from build123d import *

# Parameters (mm, degrees)
SKETCH_1_W           = 40
SKETCH_1_H           = 40
EXTRUDE_1_DEPTH      = 8
SKETCH_2_W           = 8
SKETCH_2_H           = 40
CUT_EXTRUDE_1_DEPTH  = 3.5
SKETCH_3_R           = 1.15
CUT_EXTRUDE_2_DEPTH  = 58.131427428
SKETCH_4_R           = 2
CUT_EXTRUDE_3_DEPTH  = 2.4
SKETCH_5_W           = 14.5
SKETCH_5_H           = 16
CUT_EXTRUDE_4_DEPTH  = 4
FILLET_2_R           = 0.5
SKETCH_6_W           = 1.5
SKETCH_6_H           = 1.5
CUT_EXTRUDE_5_DEPTH  = 4
SKETCH_7_R           = 1
CUT_EXTRUDE_6_DEPTH  = 4
FILLET_3_R           = 0.75
FILLET_4_R           = 0.75
CUT_EXTRUDE_7_DEPTH  = 4
SKETCH_10_R          = 3.6
CUT_EXTRUDE_9_DEPTH  = 4.5
SKETCH_11_R          = 2.1
CUT_EXTRUDE_10_DEPTH = 57.747246629


with BuildPart() as part:
    # 草图1 → 凸台-拉伸1 (new body)
    with BuildSketch(Plane(origin=(0, 0, 0), x_dir=(1, 0, 0), z_dir=(0, 1, 0))):
        with Locations((20, -20)):
            Rectangle(SKETCH_1_W, SKETCH_1_H)
    extrude(amount=EXTRUDE_1_DEPTH)

    # 草图2 → 切除-拉伸1 (cut)
    with BuildSketch(Plane(origin=(0, 8, 0), x_dir=(1, 0, 0), z_dir=(0, 1, 0))):
        with Locations((20, -20)):
            Rectangle(SKETCH_2_W, SKETCH_2_H)
    extrude(amount=-CUT_EXTRUDE_1_DEPTH, mode=Mode.SUBTRACT)

    # 草图3 → 切除-拉伸2 (cut, through all)
    with BuildSketch(Plane(origin=(0, 0, 0), x_dir=(-1, 0, 0), z_dir=(0, -1, 0))):
        with Locations(Location((-20, -30.8, 0), (0, 0, 90))):
            Circle(SKETCH_3_R)
        with Locations(Location((-20, -25.8, 0), (0, 0, 90))):
            Circle(SKETCH_3_R)
    extrude(amount=-CUT_EXTRUDE_2_DEPTH, mode=Mode.SUBTRACT)

    # 草图4 → 切除-拉伸3 (cut)
    with BuildSketch(Plane(origin=(0, 0, 0), x_dir=(-1, 0, 0), z_dir=(0, -1, 0))):
        with Locations(Location((-20, -30.8, 0), (0, 0, 90))):
            Circle(SKETCH_4_R)
        with Locations(Location((-20, -25.8, 0), (0, 0, 90))):
            Circle(SKETCH_4_R)
    extrude(amount=-CUT_EXTRUDE_3_DEPTH, mode=Mode.SUBTRACT)

    # 草图5 → 切除-拉伸4 (cut)
    with BuildSketch(Plane(origin=(0, 8, 0), x_dir=(1, 0, 0), z_dir=(0, 1, 0))):
        with Locations((8.75, -30.3)):
            Rectangle(SKETCH_5_W, SKETCH_5_H)
    extrude(amount=-CUT_EXTRUDE_4_DEPTH, mode=Mode.SUBTRACT)

    # 圆角2
    fillet_2_edges = [part.edges().sort_by_distance(p)[0] for p in [
        (16, 4.25, 22.3),
        (16, 4.25, 38.3),
        (1.5, 6, 38.3),
        (1.5, 6, 22.3),
    ]]
    fillet(fillet_2_edges, radius=FILLET_2_R)

    # 草图6 → 切除-拉伸5 (cut)
    with BuildSketch(Plane(origin=(0, 8, 0), x_dir=(1, 0, 0), z_dir=(0, 1, 0))):
        with Locations((0.75, -34.55)):
            Rectangle(SKETCH_6_W, SKETCH_6_H)
        with Locations((0.75, -30.05)):
            Rectangle(SKETCH_6_W, SKETCH_6_H)
    extrude(amount=-CUT_EXTRUDE_5_DEPTH, mode=Mode.SUBTRACT)

    # 草图7 → 切除-拉伸6 (cut)
    with BuildSketch(Plane(origin=(0, 4, 0), x_dir=(1, 0, 0), z_dir=(0, 1, 0))):
        with Locations(Location((4.5, -25.3, 0), (0, 0, 270))):
            Circle(SKETCH_7_R)
        with Locations(Location((13, -35.3, 0), (0, 0, 270))):
            Circle(SKETCH_7_R)
    extrude(amount=-CUT_EXTRUDE_6_DEPTH, mode=Mode.SUBTRACT)

    # 圆角3
    # the kernel refuses this fillet: 0.75 mm, written as the material it adds along each edge
    with BuildSketch(Plane(origin=(0, 4, 29.3), x_dir=(0, 0, 1), z_dir=(1, 0, 0)), Plane(origin=(1.5, 4, 30.8), x_dir=(0, 0, -1), z_dir=(-1, 0, 0))) as fillet_3_piece_1:
        with BuildLine():
            CenterArc((FILLET_3_R, -FILLET_3_R), FILLET_3_R, 90, 90)
            Line((0, -FILLET_3_R), (0, 0))
            Line((0, 0), (FILLET_3_R, 0))
        make_face()
    extrude(amount=1.5)

    # 圆角4
    # the kernel refuses this fillet: 0.75 mm, written as the material it adds along each edge
    with BuildSketch(Plane(origin=(0, 4, 33.8), x_dir=(0, 0, 1), z_dir=(1, 0, 0)), Plane(origin=(1.5, 4, 35.3), x_dir=(0, 0, -1), z_dir=(-1, 0, 0))) as fillet_4_piece_1:
        with BuildLine():
            CenterArc((FILLET_4_R, -FILLET_4_R), FILLET_4_R, 90, 90)
            Line((0, -FILLET_4_R), (0, 0))
            Line((0, 0), (FILLET_4_R, 0))
        make_face()
    extrude(amount=1.5)

    # 草图8 → 切除-拉伸7 (cut)
    with BuildSketch(Plane(origin=(0, 8, 0), x_dir=(1, 0, 0), z_dir=(0, 1, 0))):
        with BuildLine():
            Line((7.5, 0.415504674), (7.5, -29.155940237))
            ThreePointArc((7.5, -29.155940237), (6, -30.655940237), (4.5, -29.155940237))
            Line((4.5, -29.155940237), (4.5, 0.415504674))
            ThreePointArc((4.5, 0.415504674), (6, 1.915504674), (7.5, 0.415504674))
        make_face()
    extrude(amount=-CUT_EXTRUDE_7_DEPTH, mode=Mode.SUBTRACT)

    # 草图10 → 切除-拉伸9 (cut)
    with BuildSketch(Plane(origin=(0, 8, 0), x_dir=(1, 0, 0), z_dir=(0, 1, 0))):
        with Locations(Location((31.5, -20, 0), (0, 0, 270))):
            Circle(SKETCH_10_R)
    extrude(amount=-CUT_EXTRUDE_9_DEPTH, mode=Mode.SUBTRACT)

    # 草图11 → 切除-拉伸10 (cut, through all)
    with BuildSketch(Plane(origin=(0, 3.5, 0), x_dir=(1, 0, 0), z_dir=(0, 1, 0))):
        with Locations(Location((31.5, -20, 0), (0, 0, 270))):
            Circle(SKETCH_11_R)
    extrude(amount=-CUT_EXTRUDE_10_DEPTH, mode=Mode.SUBTRACT)


solid = part.part
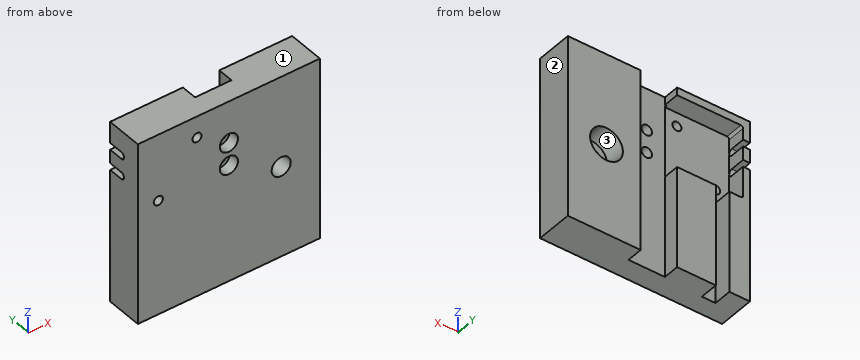
Design review of the part built by this model. Coordinates are the model's own, in mm. Face numbers are marked on the shaded views. Round coordinates to 2 decimals unless told otherwise and drop trailing zeros. Write each loop counter-clockwise with the first axis right and the second up, starting at its lowest first coordinate (ties: lowest second). Pieces come first, ordered by that corner, then holes. Notation, with made-up numbers: (-38.75, 22) -> (-27.75, 22) arc R31 ccw to (-27.75, 53) -> close; hole circle Ø1 at (19, 13.25). An arc over 180 degrees is marked (long way). One line per question, with ' | ' between items.
(1) Take a section at A-A, the plane x = 13. State the section outline as (y, z) points.
Result sheet:
outline: (0, 0) -> (8, 0) -> (8, 22.3) -> (4, 22.3) -> (4, 34.3) -> (0, 34.3) -> close; (0, 36.3) -> (4, 36.3) -> (4, 38.3) -> (8, 38.3) -> (8, 40) -> (0, 40) -> close
(2) Draft analysis for pull direction Z (two halves, no side actions). For the marked faces 1, 2 and 3, state which applies: released by +Z, released by -Z, zero draft, split by the parting line, or undercut.
Result sheet:
face 1: released by +Z | face 2: zero draft | face 3: undercut
(3) Wall thickness on line 1 (X direction, y = 6.05, z = 20); line 2 (X direction, y = 1.4, z = 35.3); line 3 (X direction, y = 2.7, z = 25.3): over which ranges is each line inside the solid? List them lowest first. Write a range as [from, to].
Result sheet:
line 1: [0, 4.5], [7.5, 16], [24, 27.9], [35.1, 40] | line 2: [0, 12], [14, 40] | line 3: [0, 3.5], [5.5, 18.96], [21.04, 40]
(4) Take a section at D-D, the plane z = 19. State the section outline as (x, y) points, and give its area (3 significant figures).
Result sheet:
outline: (0, 0) -> (29.65, 0) -> (29.65, 3.5) -> (28.04, 3.5) -> (28.04, 8) -> (24, 8) -> (24, 4.5) -> (16, 4.5) -> (16, 8) -> (7.5, 8) -> (7.5, 4) -> (4.5, 4) -> (4.5, 8) -> (0, 8) -> close; (33.35, 0) -> (40, 0) -> (40, 8) -> (34.96, 8) -> (34.96, 3.5) -> (33.35, 3.5) -> close | area: 236 mm2
(5) Take a section at C-C, the plane z = 37. State the section outline as (x, y) points, and give its area (3 significant figures).
Result sheet:
outline: (0, 0) -> (40, 0) -> (40, 8) -> (24, 8) -> (24, 4.5) -> (16, 4.5) -> (16, 4) -> (1.5, 4) -> (1.5, 8) -> (0, 8) -> close | area: 234 mm2
(6) Take a section at B-B, the plane y = 7.5. State the section outline as (x, z) points, and give its area (3 significant figures).
Result sheet:
outline: (0, 0) -> (4.5, 0) -> (4.5, 22.3) -> (2, 22.3) arc R0.5 cw to (1.5, 22.8) -> (1.5, 29.3) -> (0, 29.3) -> close; (0, 30.8) -> (1.5, 30.8) -> (1.5, 33.8) -> (0, 33.8) -> close; (0, 35.3) -> (1.5, 35.3) -> (1.5, 37.8) arc R0.5 cw to (2, 38.3) -> (16, 38.3) -> (16, 40) -> (0, 40) -> close; (7.5, 0) -> (16, 0) -> (16, 22.3) -> (7.5, 22.3) -> close; (24, 0) -> (40, 0) -> (40, 40) -> (24, 40) -> close; hole circle Ø7.2 at (31.5, 20) | area: 936 mm2
(7) Insertion check: P1, Ø5, axis at x = 4.5, z = 35, coming from the +Y side; P2, Ø3.5, axis at x = 31, z = 20.5, coming from the +Y side; P3, Ø3.5, axis at x = 20, z = 30.8, coming from the -Y side. Each pin has a flat end and moves straight along its axis. Give the tip position at first contact, or say it passes through.
Result sheet:
P1: y = 4 | P2: y = 3.5 | P3: y = 2.4
